from build123d import *

# Parameters (mm, degrees)
SKETCH1_W           = 9
SKETCH1_H           = 10
BOSS_EXTRUDE1_DEPTH = 0.4
BOSS_EXTRUDE2_DEPTH = 5
SKETCH4_W           = 0.8
SKETCH4_H           = 10
BOSS_EXTRUDE3_DEPTH = 5
CHAMFER1_SIZE       = 0.4


with BuildPart() as part:
    # Sketch1 → Boss-Extrude1 (new body)
    with BuildSketch(Plane.XY):
        with Locations((4.5, 5)):
            Rectangle(SKETCH1_W, SKETCH1_H)
    extrude(amount=BOSS_EXTRUDE1_DEPTH)

    # Sketch3 → Boss-Extrude2 (add)
    with BuildSketch(Plane.XY.offset(0.4)):
        with BuildLine():
            Line((3.5, 2), (3.5, 8.4))
            ThreePointArc((3.5, 8.4), (4.5, 9.4), (5.5, 8.4))
            Line((5.5, 8.4), (5.5, 2))
            ThreePointArc((5.5, 2), (4.5, 1), (3.5, 2))
        make_face()
    extrude(amount=BOSS_EXTRUDE2_DEPTH)

    # Sketch4 → Boss-Extrude3 (add)
    with BuildSketch(Plane.XY.offset(0.4)):
        with Locations((0.4, 5)):
            Rectangle(SKETCH4_W, SKETCH4_H)
    extrude(amount=BOSS_EXTRUDE3_DEPTH)

    # Chamfer1
    chamfer1_edges = [part.edges().sort_by_distance(p)[0] for p in [
        (4.5, 1, 5.4),
        (5.5, 5.2, 5.4),
        (4.5, 9.4, 5.4),
        (3.5, 5.2, 5.4),
    ]]
    chamfer(chamfer1_edges, length=CHAMFER1_SIZE)


solid = part.part
Read the model definition and answer for the solid it produces. Units are mm, in the model's axes. A direction names the side the tool comes from. Give positions to 0.01 mm unless a question says otherwise; leave off trailing zeros. Write each loop counter-clockwise with the first axis right and the second up, starting at its lowest first coordinate (ties: lowest second). Pieces come first, ordered by that corner, then holes. Notation, with made-up numbers: (43, 51) - (88, 51) arc R34 ccw to (88, 85) - close; hole circle Ø4 at (-39.75, 17.5). An arc over 180 degrees is marked (long way). Use CSV: the item, a comma, the result in double quotes. Start each with the question number.
Item 1: The part is cut by section B-B, the plane x = 4.5. Give the vertices of the cut face in (y, z).
Item 2: Flat-ended cylindrical pins translate along their axes: P1, Ø4, axis at x = 6, y = 3, coming from the -Z side; P2, Ø2, axis at x = 6, z = 1.5, coming from the -Y side; P3, Ø2.5, axis at y = 5, z = 3, coming from the +X side. Find the tip coordinate at first contact, or state that the pin passes through.
Item 3: The part is cut by section A-A, the plane z = 1.3. Give the vertices of the cut face in (x, y), and give its area (3 significant figures).
Item 4: The mould has two halves that part along X. Classify faces 6 (the flat face through (4.5, 5.3, 5.4)), 7 (the conical face through (4.48, 9.11, 5.29)), 8 (the flat face through (0, 5, 3)): pulls with the +X half, pulls with the -X half, needs draft (parallel to the pull), parting line crosses it, or undercut.
Item 5: Consider line 1 (X direction, y = 4.75, z = 0.75); line 2 (Z direction, x = 7, y = 4.5); line 3 (X direction, y = 1.5, z = 4.3). Determine where each line is inside the solid, lowest interval first.
Item 6: For faces 1 (the flat face through (4, 5, 0)), 2 (the flat face through (5.5, 5, 3)), 3 (the cylindrical face through (4.5, 1, 2.7)), 4 (the flat face through (0.8, 5, 3)), 5 (the cylindrical face through (4.5, 9.4, 2.7)), determine the directions among +Z, -Z, +X, -X, +Y, -Y from which every point of the face is accessible in a straight line to the end or side of a thin tool.
Item 7: The part is cut by section C-C, the plane x = 6.75. Give the vertices of the cut face in (y, z).
Taken from the geometry:
1,outline,"(0, 0) - (10, 0) - (10, 0.4) - (9.4, 0.4) - (9.4, 5) - (9, 5.4) - (1.4, 5.4) - (1, 5) - (1, 0.4) - (0, 0.4) - close"
2,P1,"z = 0"
2,P2,"y = 1.13"
2,P3,"x = 5.5"
3,outline,"(0, 0) - (0.8, 0) - (0.8, 10) - (0, 10) - close; (3.5, 2) arc R1 ccw to (5.5, 2) - (5.5, 8.4) arc R1 ccw to (3.5, 8.4) - close"
3,area,"23.9 mm2"
4,face 6,"needs draft"
4,face 7,"undercut"
4,face 8,"pulls with the -X half"
5,line 1,"0 to 0.8, 3.5 to 5.5"
5,line 2,"0 to 0.4"
5,line 3,"0 to 0.8, 3.63 to 5.37"
6,face 1,"-Z, +X, -X, +Y, -Y"
6,face 2,"+Z, +X, +Y, -Y"
6,face 3,"+Z, -Y"
6,face 4,"+Z, +Y, -Y"
6,face 5,"+Z, +Y"
7,outline,"(0, 0) - (10, 0) - (10, 0.4) - (0, 0.4) - close"
